Check sheet for the modelled part. Datum: model origin and axes. Units: mm. A direction names the side the tool comes from. Give positions to 0.01 mm unless a question says otherwise; leave off trailing zeros. Order: outer loops, then holes, each group sorted by start corner. A loop starts at its lowest first (then second) coordinate and runs counter-clockwise, first axis right, second up. Notation, with made-up numbers: (30.5, -3) - (77.5, -3) arc R21 cw to (77.5, 21) - close; hole circle Ø11 at (40.5, -10.5). An arc over 180 degrees is marked (long way). Answer in a Markdown table with one row per item.
from build123d import *

# Parameters (mm, degrees)
SKETCH_1_W          = 79
SKETCH_1_H          = 43
EXTRUDE_1_DEPTH     = 1.5
SKETCH_2_W          = 71
SKETCH_2_H          = 39
EXTRUDE_2_DEPTH     = 10.5
SKETCH_3_W          = 67
SKETCH_3_H          = 30
CUT_EXTRUDE_1_DEPTH = 8
SKETCH_4_W          = 58
SKETCH_4_H          = 23
CUT_EXTRUDE_2_DEPTH = 5
SKETCH_6_R          = 1
CUT_EXTRUDE_3_DEPTH = 9
CUT_EXTRUDE_3_TAPER = 4
SKETCH_7_R          = 1
CUT_EXTRUDE_4_DEPTH = 3
CUT_EXTRUDE_4_TAPER = 4
CUT_EXTRUDE_5_DEPTH = 3
FILLET_1_R          = 1
SKETCH_9_W          = 25
SKETCH_9_H          = 3.5
CUT_EXTRUDE_6_DEPTH = 1.5
FILLET_2_R          = 1
EXTRUDE_3_DEPTH     = 5.5


with BuildPart() as part:
    # Эскиз1 → Бобышка-Вытянуть1 (new body)
    with BuildSketch(Plane.XY):
        Rectangle(SKETCH_1_W, SKETCH_1_H)
    extrude(amount=EXTRUDE_1_DEPTH)

    # Эскиз2 → Бобышка-Вытянуть2 (add)
    with BuildSketch(Plane.XY.offset(1.5)):
        Rectangle(SKETCH_2_W, SKETCH_2_H)
    extrude(amount=EXTRUDE_2_DEPTH)

    # Эскиз3 → Вырез-Вытянуть1 (cut)
    with BuildSketch(Plane.XY.offset(12)):
        Rectangle(SKETCH_3_W, SKETCH_3_H)
    extrude(amount=-CUT_EXTRUDE_1_DEPTH, mode=Mode.SUBTRACT)

    # Эскиз4 → Вырез-Вытянуть2 (cut, through all)
    with BuildSketch(Plane.XY.offset(4)):
        with Locations((0, 0.5)):
            Rectangle(SKETCH_4_W, SKETCH_4_H)
    extrude(amount=-CUT_EXTRUDE_2_DEPTH, mode=Mode.SUBTRACT)

    # Эскиз6 → Вырез-Вытянуть3 (cut)
    with BuildSketch(Plane.XY.offset(12)):
        with Locations((-26, -17)):
            Circle(SKETCH_6_R)
        with Locations((0, -17)):
            Circle(SKETCH_6_R)
        with Locations((26, -17)):
            Circle(SKETCH_6_R)
        with Locations((20, 17)):
            Circle(SKETCH_6_R)
        with Locations((-20, 17)):
            Circle(SKETCH_6_R)
    extrude(amount=-CUT_EXTRUDE_3_DEPTH, taper=CUT_EXTRUDE_3_TAPER, mode=Mode.SUBTRACT)

    # Эскиз7 → Вырез-Вытянуть4 (cut)
    with BuildSketch(Plane.XY.offset(4)):
        with Locations((-31.5, 1)):
            Circle(SKETCH_7_R)
    cut_extrude_4 = extrude(amount=-CUT_EXTRUDE_4_DEPTH, taper=CUT_EXTRUDE_4_TAPER, mode=Mode.SUBTRACT)

    # Зеркальное отражение1: Вырез-Вытянуть4 across plane
    add(cut_extrude_4.mirror(Plane(origin=(0, 0, 0), x_dir=(0, 0, 1), z_dir=(1, 0, 0))), mode=Mode.SUBTRACT)

    # Эскиз8 → Вырез-Вытянуть5 (cut)
    with BuildSketch(Plane.XY.offset(12)):
        with BuildLine():
            Line((-17.5, 17), (17.5, 17))
            ThreePointArc((17.5, 17), (20, 14.5), (22.5, 17))
            Line((22.5, 17), (33.5, 17))
            Line((33.5, 17), (33.5, 15))
            Line((33.5, 15), (33.5, -15))
            Line((33.5, -15), (33.5, -17))
            Line((33.5, -17), (28.5, -17))
            ThreePointArc((28.5, -17), (26, -14.5), (23.5, -17))
            Line((23.5, -17), (2.5, -17))
            ThreePointArc((2.5, -17), (0, -14.5), (-2.5, -17))
            Line((-2.5, -17), (-23.5, -17))
            ThreePointArc((-23.5, -17), (-26, -14.5), (-28.5, -17))
            Line((-28.5, -17), (-33.5, -17))
            Line((-33.5, -17), (-33.5, -15))
            Line((-33.5, -15), (-33.5, 15))
            Line((-33.5, 15), (-33.5, 17))
            Line((-33.5, 17), (-22.5, 17))
            ThreePointArc((-22.5, 17), (-20, 14.5), (-17.5, 17))
        make_face()
    extrude(amount=-CUT_EXTRUDE_5_DEPTH, mode=Mode.SUBTRACT)

    # Скругление1
    fillet_1_edges = [part.edges().sort_by_distance(p)[0] for p in [
        (28.5, -17, 10.5),
        (2.5, -17, 10.5),
        (-23.5, -17, 10.5),
        (-33.5, -17, 10.5),
        (-22.5, 17, 10.5),
        (-17.5, 17, 10.5),
        (17.5, 17, 10.5),
        (22.5, 17, 10.5),
        (33.5, 17, 10.5),
        (33.5, -17, 10.5),
        (23.5, -17, 10.5),
        (-2.5, -17, 10.5),
        (-28.5, -17, 10.5),
        (-33.5, 17, 10.5),
        (-33.5, 15, 6.5),
        (33.5, 15, 6.5),
        (33.5, -15, 6.5),
        (-33.5, -15, 6.5),
    ]]
    fillet(fillet_1_edges, radius=FILLET_1_R)

    # Эскиз9 → Вырез-Вытянуть6 (cut)
    with BuildSketch(Plane.XY.offset(4)):
        with Locations((-16.5, -12.75)):
            Rectangle(SKETCH_9_W, SKETCH_9_H)
    extrude(amount=-CUT_EXTRUDE_6_DEPTH, mode=Mode.SUBTRACT)

    # Скругление2
    fillet_2_edges = [part.edges().sort_by_distance(p)[0] for p in [
        (-29, -14.5, 3.25),
        (-4, -14.5, 3.25),
    ]]
    fillet(fillet_2_edges, radius=FILLET_2_R)

    # Эскиз14 → Бобышка-Вытянуть3 (add, symmetric)
    with BuildSketch(Plane(origin=(0, 0, 0), x_dir=(1, 0, 0), z_dir=(0, 1, 0))):
        Polygon((-35.5, -1.5), (-37.5, -1.5), (-37.5, -2), (-38, -3.37373871), (-37.5, -5), (-36.245480955, -4.997017038), (-36.734683372, -3.405875127), (-36.372368855, -2.410424172), (-35.5, -2), align=None)
    extrude_3 = extrude(amount=EXTRUDE_3_DEPTH, both=True)

    # Зеркальное отражение2: Бобышка-Вытянуть3 across plane
    add(extrude_3.mirror(Plane(origin=(0, 0, 0), x_dir=(0, 0, 1), z_dir=(1, 0, 0))))


solid = part.part
(1) Cross-section at D-D, the plane y = -12.5. Record the cut outline in (x, z).
Geometry says:
| item | result |
|---|---|
| outline | (-39.5, 0) - (39.5, 0) - (39.5, 1.5) - (35.5, 1.5) - (35.5, 12) - (33.5, 12) - (33.5, 4) - (-4, 4) - (-4, 2.5) - (-29, 2.5) - (-29, 4) - (-33.5, 4) - (-33.5, 12) - (-35.5, 12) - (-35.5, 1.5) - (-39.5, 1.5) - close |
(2) Thickness scan on L1, parallel to X at y = 3, z = 9.5; L2, parallel to Y at x = -16.5, z = 3.75; L3, parallel to Y at x = 6.5, z = 5.25. Record the ranges inside material, lowest first.
Geometry says:
| item | result |
|---|---|
| L1 | -35.5 to -33.5, 33.5 to 35.5 |
| L2 | -19.5 to -14.5, 12 to 19.5 |
| L3 | -19.5 to -15, 15 to 19.5 |
(3) Cross-section at C-C, the plane x = 31.5. Record the cut outline in (y, z), then the cut area to 3 significant figures.
Geometry says:
| item | result |
|---|---|
| outline | (-21.5, 0) - (21.5, 0) - (21.5, 1.5) - (19.5, 1.5) - (19.5, 12) - (17, 12) - (17, 9) - (15, 9) - (15, 4) - (2, 4) - (1.79, 1) - (0.21, 1) - (0, 4) - (-15, 4) - (-15, 9) - (-17, 9) - (-17, 12) - (-19.5, 12) - (-19.5, 1.5) - (-21.5, 1.5) - close |
| area | 217 mm² |
(4) Access from +Z, -Z, +X, -X, +Y, -Y to the whole of each face (thin tool, end or side, straight path). Record for faces 4 (the flat face through (-36.487, 0.077, 4.213)), 5 (the flat face through (28, 17, 11)), 6 (the flat face through (39.5, 0, 1)), 7 (the flat face through (-1, 21.5, 1)), 8 (the flat face through (37.746, 0.077, 2.677)).
Geometry says:
| item | result |
|---|---|
| face 4 | +Y, -Y |
| face 5 | +Z |
| face 6 | +Z, -Z, +X, +Y, -Y |
| face 7 | +Z, -Z, +X, -X, +Y |
| face 8 | +X, +Y, -Y |
(5) Mould release check, pull along Y, two halves, no side actions. Record for faces 1 (the flat face through (37.754, 0.077, 4.175)), 2 (the conical face through (-32.21, 0.46, 2.48)), 3 (the flat face through (0, 19.5, 7)): pulls with the +Y half, pulls with the -Y half, needs draft (parallel to the pull), parting line crosses it, or undercut.
Geometry says:
| item | result |
|---|---|
| face 1 | needs draft |
| face 2 | undercut |
| face 3 | pulls with the +Y half |
(6) Cross-section at A-A, the plane x = 8. Record the cut outline in (y, z).
Geometry says:
| item | result |
|---|---|
| outline | (-21.5, 0) - (-11, 0) - (-11, 4) - (-15, 4) - (-15, 9) - (-17, 9) - (-17, 12) - (-19.5, 12) - (-19.5, 1.5) - (-21.5, 1.5) - close; (12, 0) - (21.5, 0) - (21.5, 1.5) - (19.5, 1.5) - (19.5, 12) - (17, 12) - (17, 9) - (15, 9) - (15, 4) - (12, 4) - close |
(7) Gauge pin test, flat ends, axial feed: P1, Ø1.5, axis at x = 31, z = 11, coming from the +Y side; P2, Ø1, axis at y = -3.5, z = 7.5, coming from the -X side; P3, Ø5, axis at x = 15.5, z = 8, coming from the -Y side. Record the tip position at first contact, or that the pin passes through.
Geometry says:
| item | result |
|---|---|
| P1 | y = 19.5 |
| P2 | x = -35.5 |
| P3 | y = -19.5 |
